Source: CAD feature listing. Evaluate the final solid. Frame: model axes, mm. A direction names the side the tool comes from. Coordinates: 2 decimals unless noted, no trailing zeros. Loops run counter-clockwise (first coordinate to the right, second up) from the corner with the lowest first, then second, coordinate; pieces in that order, holes last. Notation, with made-up numbers: (-11.75, 72) -> (24.25, 72) arc R25 ccw to (24.25, 95) -> close; hole circle Ø9 at (81, -9.75). An arc over 180 degrees is marked (long way). Answer as CSV lines item,"result".
Autodesk Inventor part; units mm, degrees
ref_plane "YZ Plane" through (0, 0, 0) normal (1, 0, 0) x (0, 1, 0)
ref_plane "XZ Plane" through (0, 0, 0) normal (0, 1, 0) x (-1, 0, 0)
ref_plane "XY Plane" through (0, 0, 0) normal (0, 0, 1) x (1, 0, 0)
sketch "Sketch1" plane through (0, 0, 0) normal (0, 1, 0) x (-1, 0, 0)
  line L0 (0, 0) -> (50, 0)
  line L1 (50, 0) -> (50, -80)
  line L2 (50, -80) -> (0, -80)
  line L3 (0, -80) -> (0, 0)
  dimension "d0" = 80
  dimension "d1" = 50
extrude "Extrusion1" add sketch "Sketch1" along normal blind 20
sketch "Sketch2" plane through (-50, 0, 0) normal (0, 0, 1) x (1, 0, 0)
  line L0 (5.545, 4.5622) -> (43.9524, 4.5622)
  line L1 (43.9524, 4.5622) -> (43.9524, 14.3232)
  line L2 (43.9524, 14.3232) -> (5.545, 14.3232)
  line L3 (5.545, 14.3232) -> (5.545, 4.5622)
  point P0 (50, 0)
extrude "Extrusion2" add sketch "Sketch2" along normal blind 20
sketch "Sketch3" plane through (0, 0, -80) normal (0, 0, -1) x (-1, 0, 0)
  line L0 (44.455, 14.3232) -> (6.0476, 14.3232)
  line L1 (6.0476, 4.5622) -> (44.455, 4.5622)
  line L2 (44.455, 14.3232) -> (6.0476, 14.3232)
  line L3 (6.0476, 14.3232) -> (6.0476, 4.5622)
  line L4 (6.0476, 4.5622) -> (44.455, 4.5622)
  line L5 (44.455, 4.5622) -> (44.455, 14.3232)
  point P0 (0, 0)
  point P1 (6.0476, 14.3232)
extrude "Extrusion3" add sketch "Sketch3" along normal blind 20
sketch "Sketch4" plane through (0, 0, -100) normal (0, 0, -1) x (-1, 0, 0)
  circle A0 centre (25.2513, 9.8671) radius 4.9412
  point P0 (0, 0)
extrude "Extrusion4" add sketch "Sketch4" along normal blind 25
sketch "Sketch5" plane through (-50, 0, 20) normal (0, 0, 1) x (1, 0, 0)
  circle A0 centre (24.7487, 9.6549) radius 4.9458
  point P0 (50, 0)
extrude "Extrusion5" add sketch "Sketch5" along normal blind 25
sketch "Sketch6" plane through (0, 20, 0) normal (0, 1, 0) x (1, 0, 0)
  line L0 (-33.19, 13.0471) -> (-33.19, 67.4667) construction
  line L1 (-33.19, 67.4667) -> (-19.8135, 67.4667) construction
  line L2 (-19.8135, 67.4667) -> (-19.8135, 13.0471) construction
  line L3 (-19.8135, 13.0471) -> (-33.19, 13.0471) construction
  point P0 (0, 0)
properties part number "tilt now"
(1) Cut plane D-D (y = 18.5). Return the cut outline in (x, z), then the cut area to 3 significant figures.
Computed values:
outline,"(-50, -80) -> (0, -80) -> (0, 0) -> (-50, 0) -> close"
area,"4,000 mm^2"
(2) Cut plane C-C (x = -46). Return the cut outline in (y, z).
Computed values:
outline,"(0, -80) -> (20, -80) -> (20, 0) -> (0, 0) -> close"
(3) Cut plane A-A (x = -37.5). Return the cut outline in (y, z).
Computed values:
outline,"(0, -80) -> (4.56, -80) -> (4.56, -100) -> (14.32, -100) -> (14.32, -80) -> (20, -80) -> (20, 0) -> (14.32, 0) -> (14.32, 20) -> (4.56, 20) -> (4.56, 0) -> (0, 0) -> close"
(4) Material intervals for L1, parallel to Z at x = -28, y = 19; L2, parallel to Z at x = -17, y = 12.75; L3, parallel to Y at x = -19, z = 13.5, sorted ascending. Write a range as [from, to].
Computed values:
L1,"[-80, 0]"
L2,"[-100, 20]"
L3,"[4.56, 14.32]"
(5) Cut plane B-B (y = 6.75). Return the cut outline in (x, z) (3 decimals).
Computed values:
outline,"(-50, -80) -> (-44.455, -80) -> (-44.455, -100) -> (-29.085, -100) -> (-29.085, -125) -> (-21.417, -125) -> (-21.417, -100) -> (-6.048, -100) -> (-6.048, -80) -> (0, -80) -> (0, 0) -> (-6.048, 0) -> (-6.048, 20) -> (-21.248, 20) -> (-21.248, 45) -> (-29.254, 45) -> (-29.254, 20) -> (-44.455, 20) -> (-44.455, 0) -> (-50, 0) -> close"
(6) Pin query (flat end, axial travel): pin 1 Ø12 at (x, z) = (-42, 26.5) entering from +Y; pin 2 Ø10 at (x, z) = (-16.5, 12.5) entering from +Y; pin 3 Ø2 at (y, z) = (6.5, 23.5) entering from -X; pin 4 Ø10 at (x, y) = (-14.5, 13) entering from +Z. Return the tip coordinate at first contact, or that it passes through.
Computed values:
pin 1,"through"
pin 2,"y = 14.32"
pin 3,"x = -29.7"
pin 4,"z = 20"
(7) Access query for faces 1 (the flat face through (-25, 4.562, -90)), 2 (the flat face through (-6.048, 10, -90)), 3 (the flat face through (-44.455, 10, 10)). Directions: +Z, -Z, +X, -X, +Y, -Y. A direction counts if a zero-diameter tool reaches every point of the face in a straight line with its end or side. Return the directions, or none.
Computed values:
face 1,"-Z, +X, -X, -Y"
face 2,"-Z, +X, +Y, -Y"
face 3,"+Z, -X, +Y, -Y"
